Autodesk Inventor part; units mm, degrees
ref_plane "YZ Plane" through (0, 0, 0) normal (1, 0, 0) x (0, 1, 0)
ref_plane "XZ Plane" through (0, 0, 0) normal (0, 1, 0) x (-1, 0, 0)
ref_plane "XY Plane" through (0, 0, 0) normal (0, 0, 1) x (1, 0, 0)
sketch "Boceto1" plane through (0, 0, 0) normal (0, 0, 1) x (1, 0, 0)
  line L0 (0, 0) -> (55, 0)
  line L1 (55, 0) -> (55, 20)
  line L2 (55, 20) -> (0, 20)
  line L3 (0, 20) -> (0, 0)
  circle A0 centre (6.165, 6) radius 3.5
  line L4 (27.5, 20) -> (27.5, 0)
  circle A1 centre (48.835, 6) radius 3.5
  dimension "d0" = 7
  dimension "d1" = 55
  dimension "d3" = 20
  dimension "d23" = 42.67
  dimension "d31" = 6
extrude "Extrusión1" add sketch "Boceto1" along normal blind 12
fillet "Empalme1" radius 5 2 edges at (55, 20, 6) (0, 20, 6)
sketch "Boceto7" plane through (0, 0, 0) normal (0, -1, 0) x (1, 0, 0)
  line L0 (0, 0) -> (0, 12)
  line L1 (0, 12) -> (55, 12)
  line L2 (0, 0) -> (55, 0)
  line L3 (55, 0) -> (55, 12)
  line L4 (55, 12) -> (0, 12)
  line L5 (0, 12) -> (0, 0)
extrude "Extrusión5" add sketch "Boceto7" along normal blind 10
sketch "Boceto8" plane through (55, 15, 12) normal (1, 0, 0) x (0, 0, -1)
  circle A0 centre (6, -19) radius 3.5
  line L0 (12, -25) -> (0, -25)
  line L1 (12, 0) -> (12, -25)
  point P0 (6, -25)
  dimension "d26" = 7
  dimension "d27" = 6
extrude "Extrusión6" cut sketch "Boceto8" against normal blind 55
properties part number "SoporteDerecha"
Model file for the job. Use its own axes, mm. Give positions to 0.01 mm unless a question says otherwise; leave off trailing zeros. Write each loop counter-clockwise with the first axis right and the second up, starting at its lowest first coordinate (ties: lowest second). Pieces come first, ordered by that corner, then holes. Notation, with made-up numbers: M 59,52 L 82,52 A22 cw 82,77 Z; hole C 14.25,57.25 d7. An arc over 180 degrees is marked long. One line per item, written item: value. Start each with the question number.
Q1. Saw through at A-A, the plane y = 6. Write the cut outline in (x, z) (3 decimals).
Q2. Drop a flat-ended pin along its axis: pin 1 Ø5.5 at (x, y) = (48.835, 6) entering from -Z. Give the stop position or say it passes through.
Q3. Saw through at D-D, the plane x = 48. Write the cut outline in (y, z), plus the area to 3 significant figures.
Q4. Saw through at C-C, the plane y = -4. Write the cut outline in (x, z).
Q5. Saw through at B-B, the plane z = 6. Write the cut outline in (x, y) (3 decimals), plus the area to 3 significant figures.
Q6. Probe probe 1 along Y at (x, z) = (50.5, 7.5); probe 2 along X at (y, z) = (6.25, 3.25); probe 3 along X at (y, z) = (3, 11). List the from-to ranges inside material, lowest first. Write a range as [from, to].
Q7. Two-plate mould, pull along Z, no slides. Class faces 1 (the flat face through (27, 5, 0)), 2 (the cylindrical face through (27.885, -7.417, 6.759)), 3 (the cylindrical face through (54, 18, 6)), 4 (the flat face through (27, 5, 12)): +Z half, -Z half, draft (parallel to the pull), parting line (faces both ways), or undercut.
Output values:
1. outline: M 0,0 L 2.665,0 L 2.665,12 L 0,12 Z; M 9.665,0 L 45.335,0 L 45.335,12 L 9.665,12 Z; M 52.335,0 L 55,0 L 55,12 L 52.335,12 Z
2. pin 1: passes through
3. outline: M -10,0 L 2.6,0 L 2.6,12 L -10,12 Z; M 9.4,0 L 20,0 L 20,12 L 9.4,12 Z; hole C -4,6 d7
3. area: 240 mm²
4. outline: M 0,0 L 55,0 L 55,2.5 L 0,2.5 Z; M 0,9.5 L 55,9.5 L 55,12 L 0,12 Z
5. outline: M 0,-10 L 55,-10 L 55,-7.5 L 0,-7.5 Z; M 0,-0.5 L 55,-0.5 L 55,15 A5 ccw 50,20 L 5,20 A5 ccw 0,15 Z; hole C 6.165,6 d7; hole C 48.835,6 d7
5. area: 1,180 mm²
6. probe 1: y = [-10, -7.16], [-0.84, 2.92], [9.08, 19.97]
6. probe 2: x = [0, 2.67], [9.66, 45.34], [52.33, 55]
6. probe 3: x = [0, 4.36], [7.97, 47.03], [50.64, 55]
7. face 1: -Z half
7. face 2: undercut
7. face 3: draft
7. face 4: +Z half
